```python
from build123d import *

# Parameters (mm, degrees)
SKETCH001002046_W = 37
SKETCH001002046_H = 79
PAD033_DEPTH      = 1.25
SKETCH001002042_R = 1
SKETCH001002042_W = 30
SKETCH001002042_H = 68
POCKET017_DEPTH   = 1
SKETCH001002049_W = 9.5
SKETCH001002049_H = 1
POCKET018_DEPTH   = 1
FILLET038_R       = 0.3


with BuildPart() as part:
    # Sketch001002046 → Pad033 (new body)
    with BuildSketch(Plane.XY):
        Rectangle(SKETCH001002046_W, SKETCH001002046_H)
    extrude(amount=PAD033_DEPTH)

    # Sketch001002042 → Pocket017 (cut)
    with BuildSketch(Plane.XY.offset(0.8)):
        with BuildLine():
            Line((-16, 38), (16, 38))
            Line((16, 38), (16, -35))
            Line((11, -35), (16, -35))
            Line((11, -33), (11, -35))
            ThreePointArc((11, -33), (10.707107, -32.292893), (10, -32))
            Line((-10, -32), (10, -32))
            ThreePointArc((-10, -32), (-10.707107, -32.292893), (-11, -33))
            Line((-11, -35), (-11, -33))
            Line((-16, -35), (-11, -35))
            Line((-16, -35), (-16, 38))
        make_face()
        with Locations((-13.5, -33)):
            Circle(SKETCH001002042_R, mode=Mode.SUBTRACT)
        with Locations((13.5, -33)):
            Circle(SKETCH001002042_R, mode=Mode.SUBTRACT)
        with Locations((0, 3)):
            Rectangle(SKETCH001002042_W, SKETCH001002042_H, mode=Mode.SUBTRACT)
    extrude(amount=POCKET017_DEPTH, mode=Mode.SUBTRACT)

    # Sketch001002049 → Pocket018 (cut)
    with BuildSketch(Plane.XY.offset(0.8)):
        with BuildLine():
            Line((-18.5, -39.5), (18.5, -39.5))
            Line((18.5, -39.5), (18.5, -36.5))
            Line((18.5, -36.5), (10.5, -36.5))
            Line((10.5, -36.5), (10.5, -33.5))
            ThreePointArc((10.5, -33.5), (10.207107, -32.792893), (9.5, -32.5))
            Line((9.5, -32.5), (-9.5, -32.5))
            Line((-9.5, -32.5), (-10.5, -36.5))
            Line((-10.5, -36.5), (-18.5, -36.5))
            Line((-18.5, -36.5), (-18.5, -39.5))
        make_face()
        with Locations((0, -37)):
            Rectangle(SKETCH001002049_W, SKETCH001002049_H, mode=Mode.SUBTRACT)
    extrude(amount=POCKET018_DEPTH, mode=Mode.SUBTRACT)

    # Fillet038
    fillet038_edges = [part.edges().sort_by_distance(p)[0] for p in [
        (0, 39.5, 1.25),
        (-18.5, 1.5, 1.25),
        (18.5, 1.5, 1.25),
    ]]
    fillet(fillet038_edges, radius=FILLET038_R)


solid = part.part
```
Here's how the part is built. I have some questions about the finished solid (model axes, mm). A direction names the side the tool comes from. Give positions to 0.01 mm unless a question says otherwise; leave off trailing zeros. Write each loop counter-clockwise with the first axis right and the second up, starting at its lowest first coordinate (ties: lowest second). Pieces come first, ordered by that corner, then holes.
(1) On a 3-axis mill with a long thin cutter (end or side, diameter ignored), from which of +Z, -Z, +X, -X, +Y, -Y can I reach the whole of each face in a straight line? I mean faces 1 (the face through (-12.96, -32.16, 1.02)), 2 (the face through (13, -33, 1.25)). Say none if no direction works.
Output values:
face 1: +Z
face 2: +Z, +X, -X, +Y, -Y
(2) Thinking about a two-plate mould opening in X: for faces 3 (the face through (0, -36, 0.8)), 4 (the face through (14.04, -32.16, 1.02)), 5 (the face through (-14, -33, 1.25)), which applies, pulls with the +X half, pulls with the -X half, needs draft (parallel to the pull), parting line crosses it, or undercut?
Output values:
face 3: undercut
face 4: undercut
face 5: needs draft
(3) Imagine slicing it at D-D, the plane x = 5.5. Write out the boundary of the cut face in (y, z).
Output values:
outline: (-39.5, 0) - (39.5, 0) - (39.5, 0.95) arc R0.3 ccw to (39.2, 1.25) - (38, 1.25) - (38, 0.8) - (37, 0.8) - (37, 1.25) - (-31, 1.25) - (-31, 0.8) - (-32, 0.8) - (-32, 1.25) - (-32.5, 1.25) - (-32.5, 0.8) - (-39.5, 0.8) - close
(4) Imagine slicing it at C-C, the plane x = -13.5. Write out the boundary of the cut face in (y, z), and give its area (3 significant figures).
Output values:
outline: (-39.5, 0) - (39.5, 0) - (39.5, 0.95) arc R0.3 ccw to (39.2, 1.25) - (38, 1.25) - (38, 0.8) - (37, 0.8) - (37, 1.25) - (-31, 1.25) - (-31, 0.8) - (-32, 0.8) - (-32, 1.25) - (-34, 1.25) - (-34, 0.8) - (-35, 0.8) - (-35, 1.25) - (-36.5, 1.25) - (-36.5, 0.8) - (-39.5, 0.8) - close
area: 96.0 mm2
(5) Imagine slicing it at A-A, the plane x = 1. Write out the boundary of the cut face in (y, z).
Output values:
outline: (-39.5, 0) - (39.5, 0) - (39.5, 0.95) arc R0.3 ccw to (39.2, 1.25) - (38, 1.25) - (38, 0.8) - (37, 0.8) - (37, 1.25) - (-31, 1.25) - (-31, 0.8) - (-32, 0.8) - (-32, 1.25) - (-32.5, 1.25) - (-32.5, 0.8) - (-36.5, 0.8) - (-36.5, 1.25) - (-37.5, 1.25) - (-37.5, 0.8) - (-39.5, 0.8) - close
(6) If I drill on L1, parallel to Y at x = 8.5, z = 0.9; L2, parallel to X at y = -14, z = 0.9; L3, parallel to Y at x = -4.5, z = 0.9, over which ranges is the centre line in solid material (lowest first)?
Output values:
L1: y = -32.5 to -32, -31 to 37, 38 to 39.5
L2: x = -18.5 to -16, -15 to 15, 16 to 18.5
L3: y = -37.5 to -36.5, -32.5 to -32, -31 to 37, 38 to 39.5
(7) Imagine slicing it at B-B, the plane y = -3. Write out the boundary of the cut face in (x, z), and give its area (3 significant figures).
Output values:
outline: (-18.5, 0) - (18.5, 0) - (18.5, 0.95) arc R0.3 ccw to (18.2, 1.25) - (16, 1.25) - (16, 0.8) - (15, 0.8) - (15, 1.25) - (-15, 1.25) - (-15, 0.8) - (-16, 0.8) - (-16, 1.25) - (-18.2, 1.25) arc R0.3 ccw to (-18.5, 0.95) - close
area: 45.3 mm2
